```python
from build123d import *

# Parameters (mm, degrees)
TOOTH_DEPTH       = 6.35
CIRPATTERN2_COUNT = 13
FILLET1_START     = -1
FILLET1_DEPTH     = 8
CIRPATTERN4_COUNT = 13
BEARING_START     = -6.35
SKETCH2_R         = 17.145
SKETCH2_R_2       = 3.81
BEARING_DEPTH     = 6.35


with BuildPart() as part:
    # Sketch1 → tooth (new body)
    with BuildSketch(Plane(origin=(0, 0, 0), x_dir=(1, 0, 0), z_dir=(0, 1, 0))):
        with BuildLine():
            Line((20.955, 1.905), (24.430024666, 4.059448215))
            ThreePointArc((24.430024666, 4.059448215), (24.045374001, 5.92665286), (23.518231918, 7.758736523))
            Line((23.518231918, 7.758736523), (16.281852867, 5.371432977))
            ThreePointArc((16.281852867, 5.371432977), (17.094199899, 1.318846017), (16.913093955, -2.810387497))
            Line((16.913093955, -2.810387497), (24.430024666, -4.059448215))
            Line((24.430024666, -4.059448215), (20.955, -1.905))
            ThreePointArc((20.955, -1.905), (21.041412738, 0), (20.955, 1.905))
        make_face()
    tooth = extrude(amount=TOOTH_DEPTH)

    # CirPattern2: tooth ×13 about axis
    cirpattern2_axis = Axis((0, 0, 0), (0, 1, 0))
    for i in range(1, CIRPATTERN2_COUNT):
        add(tooth.rotate(cirpattern2_axis, i * 360 / CIRPATTERN2_COUNT))

    # Fillet1: read off the stored shape, not the designer's step
    # Fillet1 outline → Fillet1 (cut)
    with BuildSketch(Plane(origin=(0, 0, 0), x_dir=(1, 0, 0), z_dir=(0, 1, 0)).offset(FILLET1_START)):
        with BuildLine():
            Line((23.518231918, 7.758736523), (22.653265955, 7.820825329))
            ThreePointArc((22.653265955, 7.820825329), (23.360778925, 7.541702395), (23.781921552, 6.908359594))
            ThreePointArc((23.781921552, 6.908359594), (23.653898512, 7.334733136), (23.518231918, 7.758736523))
        make_face()
        with BuildLine():
            ThreePointArc((24.430024666, 4.059448215), (24.353107335, 4.497931535), (24.268320524, 4.934961391))
            ThreePointArc((24.268320524, 4.934961391), (24.189746323, 4.178449454), (23.692989596, 3.602500698))
            Line((23.692989596, 3.602500698), (24.430024666, 4.059448215))
        make_face()
    fillet1 = extrude(amount=FILLET1_DEPTH, mode=Mode.SUBTRACT)

    # CirPattern4: Fillet1 ×13 about axis
    cirpattern4_axis = Axis((0, 0, 0), (0, 1, 0))
    for i in range(1, CIRPATTERN4_COUNT):
        add(fillet1.rotate(cirpattern4_axis, i * 360 / CIRPATTERN4_COUNT), mode=Mode.SUBTRACT)

    # Sketch2 → bearing (add)
    with BuildSketch(Plane(origin=(0, 6.35, 0), x_dir=(1, 0, 0), z_dir=(0, 1, 0)).offset(BEARING_START)):
        Circle(SKETCH2_R)
        with Locations(Location((0, 0, 0), (0, 0, 270))):
            Circle(SKETCH2_R_2, mode=Mode.SUBTRACT)
        with Locations(Location((12.7, 0, 0), (0, 0, 270))):
            Circle(SKETCH2_R_2, mode=Mode.SUBTRACT)
        with Locations(Location((6.35, -10.998522628, 0), (0, 0, 270))):
            Circle(SKETCH2_R_2, mode=Mode.SUBTRACT)
        with Locations(Location((-6.35, -10.998522628, 0), (0, 0, 270))):
            Circle(SKETCH2_R_2, mode=Mode.SUBTRACT)
        with Locations(Location((-12.7, 0, 0), (0, 0, 270))):
            Circle(SKETCH2_R_2, mode=Mode.SUBTRACT)
        with Locations(Location((-6.35, 10.998522628, 0), (0, 0, 270))):
            Circle(SKETCH2_R_2, mode=Mode.SUBTRACT)
        with Locations(Location((6.35, 10.998522628, 0), (0, 0, 270))):
            Circle(SKETCH2_R_2, mode=Mode.SUBTRACT)
    extrude(amount=BEARING_DEPTH)


solid = part.part
```
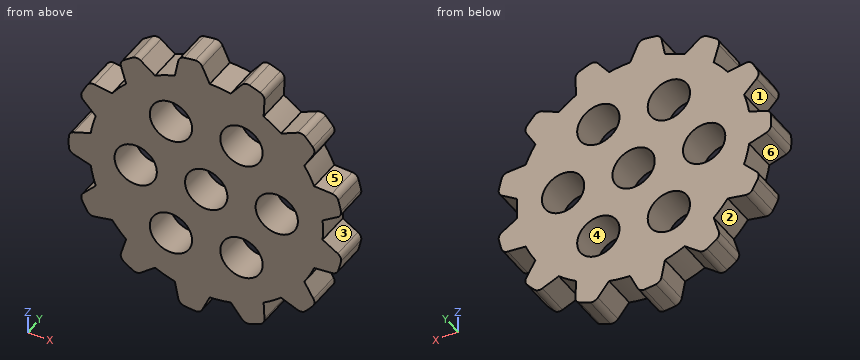
Input: part model. Units: mm. Frame: model coordinates. Face numbers are marked on the shaded views. A direction names the side the tool comes from. Give positions to 0.01 mm unless a question says otherwise; leave off trailing zeros. Order: outer loops, then holes, each group sorted by start corner. A loop starts at its lowest first (then second) coordinate and runs counter-clockwise, first axis right, second up. Notation, with made-up numbers: M -39,46.5 L -10,46.5 A22 cw -10,80.5 Z; hole C -17,76.5 d1. An arc over 180 degrees is marked long. Return JSON: item names as keys, results as strings.
1) Section query C-C on x = 0. Output: boundary loops of the cut face in (y, z), and give its area (3 significant figures).
Taken from the geometry:
{"outline": "M 0,-22.4 L 6.35,-22.4 L 6.35,-3.81 L 0,-3.81 Z; M 0,3.81 L 6.35,3.81 L 6.35,22.4 L 0,22.4 Z", "area": "236 mm2"}
2) Contact query for flat-ended pins moving along their axis: pin 1 (2 mm diameter, centred on x = -3.5, y = 3, fed in from -Z); pin 2 (9 mm diameter, centred on x = 0, z = 0, fed in from -Y); pin 3 (6 mm diameter, centred on x = -6.35, z = -11, fed in from +Y); pin 4 (3 mm diameter, centred on x = 0.5, y = 5.5, fed in from +Z). Output: stop coordinate, or through.
Taken from the geometry:
{"pin 1": "stops at z = -24.64", "pin 2": "stops at y = 0", "pin 3": "passes through", "pin 4": "stops at z = 24.34"}
3) Section query B-B on x = 7. Output: boundary loops of the cut face in (y, z).
Taken from the geometry:
{"outline": "M 0,-23.49 L 6.35,-23.49 L 6.35,-14.75 L 0,-14.75 Z; M 0,-7.24 L 6.35,-7.24 L 6.35,7.24 L 0,7.24 Z; M 0,14.75 L 6.35,14.75 L 6.35,23.49 L 0,23.49 Z"}
4) Line query: L1, parallel to X at y = 3, z = 0 (3 decimals); L2, parallel to X at y = 5.5, z = 11; L3, parallel to X at y = 5.25, z = -1. Output: solid intervals per line, ascending. Write a range as [from, to].
Taken from the geometry:
{"L1": "x = [-24.765, -16.51], [-8.89, -3.81], [3.81, 8.89], [16.51, 21.041]", "L2": "x = [-22.19, -10.16], [-2.54, 2.54], [10.16, 17.94]", "L3": "x = [-24.74, -16.38], [-9.02, -3.68], [3.68, 9.02], [16.38, 21.02]"}
5) Access query for the marked faces 1, 2 and 3. Directions: +Z, -Z, +X, -X, +Y, -Y. A direction counts if a zero-diameter tool reaches every point of the face in a straight line with its end or side. Return the directions, or none.
Taken from the geometry:
{"face 1": "-X, +Y, -Y", "face 2": "+Y, -Y", "face 3": "+X, +Y, -Y"}
6) Section query D-D on y = 1.75. Count the separate pieces of the cut face and the enclosed holes in it, and give its area (3 significant figures).
Taken from the geometry:
{"separate pieces": "1", "enclosed holes": "7", "area": "1,310 mm2"}
7) Section query A-A on z = 0. Output: boundary loops of the cut face in (x, y) (3 decimals), and give its area (3 significant figures).
Taken from the geometry:
{"outline": "M -24.765,0 L -16.51,0 L -16.51,6.35 L -24.765,6.35 Z; M -8.89,0 L -3.81,0 L -3.81,6.35 L -8.89,6.35 Z; M 3.81,0 L 8.89,0 L 8.89,6.35 L 3.81,6.35 Z; M 16.51,0 L 21.041,0 L 21.041,6.35 L 16.51,6.35 Z", "area": "146 mm2"}
8) Mould query, pull axis X, two halves, no side actions, for the marked faces 4, 5 and 6. Classes: released by +X, released by -X, zero draft, split by the parting line, or undercut.
Taken from the geometry:
{"face 4": "undercut", "face 5": "released by +X", "face 6": "released by -X"}
